Geometry: final body of the model. Coordinates: model frame, mm. A direction names the side the tool comes from. Round coordinates to 2 decimals unless told otherwise and drop trailing zeros. Loops run counter-clockwise (first coordinate to the right, second up) from the corner with the lowest first, then second, coordinate; pieces in that order, holes last. Notation, with made-up numbers: (74.25, 61.25) -> (107.25, 61.25) arc R29 ccw to (107.25, 91.25) -> close; hole circle Ø6 at (42.25, 30). An arc over 180 degrees is marked (long way). Answer in a Markdown table with one row per item.
```python
from build123d import *

# Parameters (mm, degrees)
SKETCH1_W           = 200
SKETCH1_H           = 100
BOSS_EXTRUDE1_DEPTH = 6.36
SKETCH9_W           = 6.96
SKETCH9_H           = 50
BOSS_EXTRUDE5_DEPTH = 6.36
SKETCH10_W          = 100
SKETCH10_H          = 5.76
CUT_EXTRUDE1_DEPTH  = 119.240818671
SKETCH13_R          = 2
BATTERY_HOLES_DEPTH = 10
SKETCH14_W          = 12
SKETCH14_H          = 10.5
CUT_EXTRUDE6_DEPTH  = 119.240818671


with BuildPart() as part:
    # Sketch1 → Boss-Extrude1 (new body)
    with BuildSketch(Plane.XY):
        Rectangle(SKETCH1_W, SKETCH1_H)
    extrude(amount=BOSS_EXTRUDE1_DEPTH)

    # Sketch9 → Boss-Extrude5 (add)
    with BuildSketch(Plane(origin=(0, 0, 0), x_dir=(-1, 0, 0), z_dir=(0, 0, -1))):
        with Locations((103.48, 0)):
            Rectangle(SKETCH9_W, SKETCH9_H)
    boss_extrude5 = extrude(amount=-BOSS_EXTRUDE5_DEPTH)

    # Mirror5: Boss-Extrude5 across plane
    add(boss_extrude5.mirror(Plane(origin=(0, 0, 0), x_dir=(0, 0, 1), z_dir=(1, 0, 0))))

    # Sketch10 → Cut-Extrude1 (cut, symmetric)
    with BuildSketch(Plane.XY.offset(6.36)):
        with Locations((0, 47.12)):
            Rectangle(SKETCH10_W, SKETCH10_H)
    cut_extrude1 = extrude(amount=CUT_EXTRUDE1_DEPTH, both=True, mode=Mode.SUBTRACT)

    # Mirror6: Cut-Extrude1 across plane
    add(cut_extrude1.mirror(Plane.ZX), mode=Mode.SUBTRACT)

    # Sketch13 → battery holes (cut)
    with BuildSketch(Plane.XY.offset(6.36)):
        with Locations((50, -15)):
            Circle(SKETCH13_R)
        with Locations((28.5, -1.5)):
            Circle(SKETCH13_R)
        with Locations((28.5, -28.5)):
            Circle(SKETCH13_R)
    extrude(amount=-BATTERY_HOLES_DEPTH, mode=Mode.SUBTRACT)

    # Sketch14 → Cut-Extrude6 (cut, through all)
    with BuildSketch(Plane(origin=(0, 0, 0), x_dir=(-1, 0, 0), z_dir=(0, 0, -1))):
        with Locations((39.2, -24.09)):
            Rectangle(SKETCH14_W, SKETCH14_H)
    extrude(amount=-CUT_EXTRUDE6_DEPTH, mode=Mode.SUBTRACT)


solid = part.part
```
Item 1: Pin query (flat end, axial travel): pin 1 Ø3 at (x, z) = (-41, 4) entering from +Y; pin 2 Ø3 at (x, z) = (-40, 4) entering from -Y; pin 3 Ø1.9 at (x, z) = (105, 4.5) entering from +Y. Return the tip coordinate at first contact, or that it passes through.
Answer:
| item | result |
|---|---|
| pin 1 | stops at y = 44.24 |
| pin 2 | stops at y = -44.24 |
| pin 3 | stops at y = 25 |
Item 2: Line query: probe 1 along Y at (x, z) = (28.5, 3.25); probe 2 along Y at (x, z) = (-37, 5.75); probe 3 along Y at (x, z) = (-8, 4). Output: solid intervals per line, ascending. Write a range as [from, to].
Answer:
| item | result |
|---|---|
| probe 1 | y = [-44.24, -30.5], [-26.5, -3.5], [0.5, 44.24] |
| probe 2 | y = [-44.24, -29.34], [-18.84, 44.24] |
| probe 3 | y = [-44.24, 44.24] |
Item 3: Cut plane D-D (y = 40). Output: boundary loops of the cut face in (x, z), then the cut area to 3 significant figures.
Answer:
| item | result |
|---|---|
| outline | (-100, 0) -> (100, 0) -> (100, 6.36) -> (-100, 6.36) -> close |
| area | 1,270 mm² |
Item 4: Cut plane A-A (y = -15). Output: boundary loops of the cut face in (x, z).
Answer:
| item | result |
|---|---|
| outline | (-106.96, 0) -> (48, 0) -> (48, 6.36) -> (-106.96, 6.36) -> close; (52, 0) -> (106.96, 0) -> (106.96, 6.36) -> (52, 6.36) -> close |
Item 5: Cut plane C-C (z = 3.25). Output: boundary loops of the cut face in (x, y).
Answer:
| item | result |
|---|---|
| outline | (-106.96, -25) -> (-100, -25) -> (-100, -50) -> (-50, -50) -> (-50, -44.24) -> (50, -44.24) -> (50, -50) -> (100, -50) -> (100, -25) -> (106.96, -25) -> (106.96, 25) -> (100, 25) -> (100, 50) -> (50, 50) -> (50, 44.24) -> (-50, 44.24) -> (-50, 50) -> (-100, 50) -> (-100, 25) -> (-106.96, 25) -> close; hole (-45.2, -29.34) -> (-33.2, -29.34) -> (-33.2, -18.84) -> (-45.2, -18.84) -> close; hole circle Ø4 at (28.5, -28.5); hole circle Ø4 at (28.5, -1.5); hole circle Ø4 at (50, -15) |
Item 6: Cut plane B-B (x = 28.5). Output: boundary loops of the cut face in (y, z).
Answer:
| item | result |
|---|---|
| outline | (-44.24, 0) -> (-30.5, 0) -> (-30.5, 6.36) -> (-44.24, 6.36) -> close; (-26.5, 0) -> (-3.5, 0) -> (-3.5, 6.36) -> (-26.5, 6.36) -> close; (0.5, 0) -> (44.24, 0) -> (44.24, 6.36) -> (0.5, 6.36) -> close |
Item 7: Reachability of faces 1 (the face through (100, 37, 3)), 2 (the face through (-1, -44.24, 3)), 3 (the face through (-45.2, -24, 3)), 4 (the face through (100, -38, 3)), 5 (the face through (-50, 47, 3)) from +Z, -Z, +X, -X, +Y, -Y: full face, straight path, thin tool, end or side. Return the list, or none.
Answer:
| item | result |
|---|---|
| face 1 | +Z, -Z, +X, +Y |
| face 2 | +Z, -Z, -Y |
| face 3 | +Z, -Z |
| face 4 | +Z, -Z, +X, -Y |
| face 5 | +Z, -Z, +Y |
Item 8: Draft query along Y for faces 6 (the face through (-39, -29.34, 3)), 7 (the face through (-75, 50, 3)), 8 (the face through (-75, -50, 3)), 9 (the face through (-100, 37, 3)). Return one class per face: pulls with the +Y half, pulls with the -Y half, needs draft (parallel to the pull), parting line crosses it, or undercut.
Answer:
| item | result |
|---|---|
| face 6 | undercut |
| face 7 | pulls with the +Y half |
| face 8 | pulls with the -Y half |
| face 9 | needs draft |
